Verification items for the finished model (mm, model axes). A direction names the side the tool comes from. Give positions to 0.01 mm unless a question says otherwise; leave off trailing zeros. Loops run counter-clockwise (first coordinate to the right, second up) from the corner with the lowest first, then second, coordinate; pieces in that order, holes last. Notation, with made-up numbers: (5, 65) - (44, 65) arc R13 ccw to (44, 86) - close; hole circle Ø10 at (51, -31.5). An arc over 180 degrees is marked (long way). Put each result on its own line as item: value. Start each with the question number.
```python
from build123d import *

# Parameters (mm, degrees)
SKETCH1_W           = 22
SKETCH1_H           = 22
SKETCH1_R           = 4.5
BOSS_EXTRUDE1_DEPTH = 3
SKETCH1_3_R         = 4.5
BOSS_EXTRUDE2_DEPTH = 30
SKETCH2_R           = 3
BOSS_EXTRUDE3_DEPTH = 26
FILLET1_R           = 0.5
FILLET4_R           = 0.5
FILLET5_R           = 1
CHAMFER2_SIZE       = 3
FILLET7_R           = 2


with BuildPart() as part:
    # Sketch1 → Boss-Extrude1 (new body)
    # profile 1 of 2: a face of its own
    with BuildSketch(Plane.XY):
        Rectangle(SKETCH1_W, SKETCH1_H)
        Circle(SKETCH1_R, mode=Mode.SUBTRACT)
    # profile 2 of 2: a face of its own
    with BuildSketch(Plane.XY):
        Circle(SKETCH1_R)
    extrude(amount=BOSS_EXTRUDE1_DEPTH)

    # Sketch1_3 → Boss-Extrude2 (add)
    with BuildSketch(Plane.XY):
        Circle(SKETCH1_3_R)
    extrude(amount=-BOSS_EXTRUDE2_DEPTH)

    # Sketch2 → Boss-Extrude3 (add)
    with BuildSketch(Plane(origin=(0, 0, -30), x_dir=(-1, 0, 0), z_dir=(0, 0, -1))):
        with Locations(Location((0, 0, 0), (0, 0, 180))):
            Circle(SKETCH2_R)
    extrude(amount=BOSS_EXTRUDE3_DEPTH)

    # Sketch3 → Cut-Revolve1 (revolve, cut)
    with BuildSketch(Plane(origin=(0, 0, 0), x_dir=(0, 0, -1), z_dir=(1, 0, 0)), mode=Mode.PRIVATE) as cut_revolve1_sk:
        Polygon((30, 3), (26, 4.5), (30, 4.5), align=None)
    revolve(cut_revolve1_sk.sketch.rotate(Axis((0, 0, -30), (0, 0, 1)), 270), axis=Axis((0, 0, -30), (0, 0, 1)), mode=Mode.SUBTRACT)

    # Fillet1
    fillet1_edges = [part.edges().sort_by_distance(p)[0] for p in [
        (-4.5, 0, 0),
    ]]
    fillet(fillet1_edges, radius=FILLET1_R)

    # Fillet4
    fillet4_edges = [part.edges().sort_by_distance(p)[0] for p in [
        (-3, 0, -56),
    ]]
    fillet(fillet4_edges, radius=FILLET4_R)

    # Fillet5
    fillet5_edges = [part.edges().sort_by_distance(p)[0] for p in [
        (-4.5, 0, -26),
    ]]
    fillet(fillet5_edges, radius=FILLET5_R)

    # Chamfer2
    chamfer2_edges = [part.edges().sort_by_distance(p)[0] for p in [
        (11, -11, 1.5),
        (-11, -11, 1.5),
        (-11, 11, 1.5),
        (11, 11, 1.5),
    ]]
    chamfer(chamfer2_edges, length=CHAMFER2_SIZE)

    # Fillet7
    fillet7_edges = [part.edges().sort_by_distance(p)[0] for p in [
        (-8, 11, 1.5),
        (8, 11, 1.5),
        (11, -8, 1.5),
        (11, 8, 1.5),
        (-11, -8, 1.5),
        (-11, 8, 1.5),
        (8, -11, 1.5),
        (-8, -11, 1.5),
    ]]
    fillet(fillet7_edges, radius=FILLET7_R)


solid = part.part
```
1) Section check B-B, the plane z = -3. Enter the section's corners in (x, y).
2) Section check A-A, the plane x = -6.5. Enter the section's corners in (y, z).
3) Section check C-C, the plane z = -44. Enter the section's corners in (x, y).
4) Set-up check for faces 1 (the face through (4.292, 1.352, -12.982)), 2 (the face through (10.844, -7.947, 1.521)): record each of +Z, -Z, +X, -X, +Y, -Y from which the full face is reachable in a straight line by a thin tool's end or side.
5) Scan lines: line 1 along Z through (x, y) = (-9.75, -8.25); line 2 along X through (y, z) = (0.75, -15); line 3 along Y through (x, z) = (-2, -32.5). Record each from-to range of solid material in increasing order. Write a range as from..to.
6) Depth check by flat-ended pin: P1, Ø1, axis at x = -1, z = -21, coming from the -Y side; P2, Ø8, axis at x = 8.5, y = 6.5, coming from the -Z side; P3, Ø8, axis at x = -4.5, y = -7.5, coming from the -Z side. Enter the tip coordinate at first touch or a pass-through.
Results are:
1. outline: circle Ø9 at (0, 0)
2. outline: (-11, 0) - (11, 0) - (11, 3) - (-11, 3) - close
3. outline: circle Ø6 at (0, 0)
4. face 1: -Z
4. face 2: +Z, -Z, +X, -Y
5. line 1: z = 0..3
5. line 2: x = -4.44..4.44
5. line 3: y = -2.24..2.24
6. P1: stops at y = -4.47
6. P2: stops at z = 0
6. P3: stops at z = -0.07
